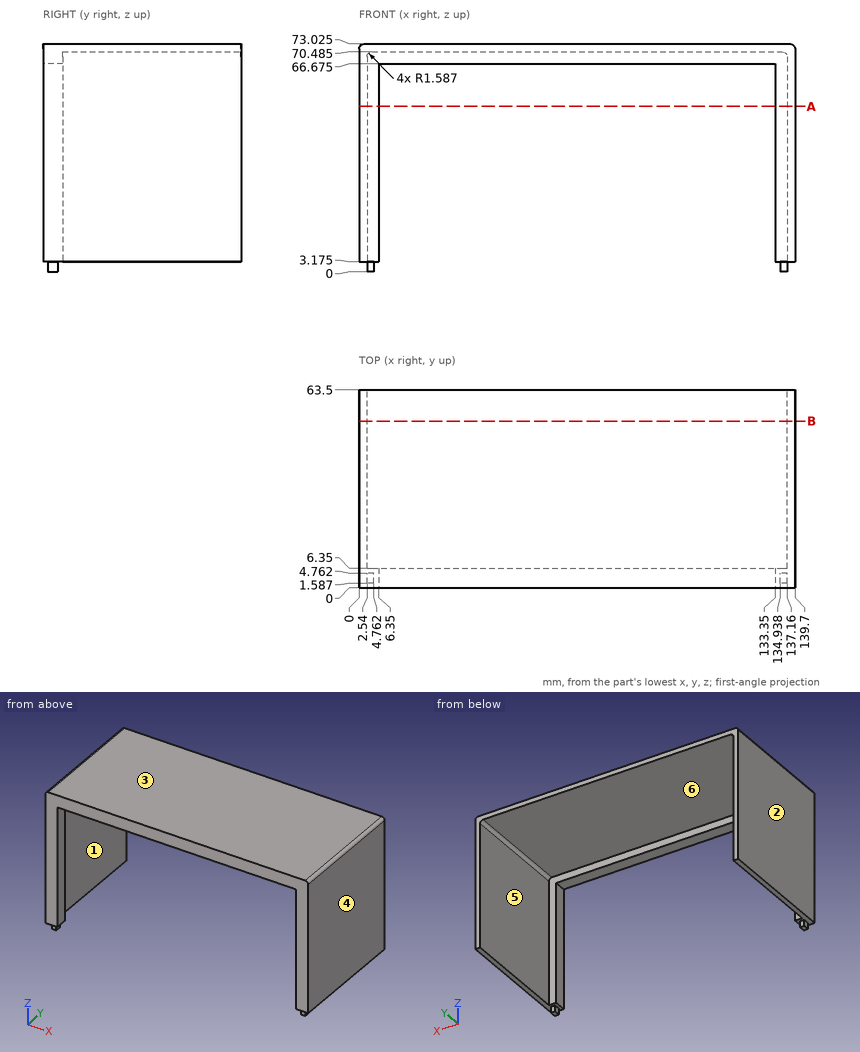
Job drawing, mm, ordinate dimensions from the low corner. One solid piece. A direction names the side the tool comes from. Round coordinates to 2 decimals unless told otherwise and drop trailing zeros. Loops run counter-clockwise (first coordinate to the right, second up) from the corner with the lowest first, then second, coordinate; pieces in that order, holes last.
Item 1: Drop flat-ended pins along their axis: P1, Ø1.6, axis at y = 3, z = 1.5, coming from the +X side; P2, Ø7, axis at x = 78.5, y = 3.5, coming from the -Z side (1 decimal); P3, Ø7, axis at x = 135.5, y = 41, coming from the -Z side (1 decimal). Give the stop position or say it passes through.
Item 2: Mould opens along X. For the marked faces 3, 4, 5 and 6 say: +X half, -X half, draft (parallel to the pull), parting line (faces both ways), or undercut.
Item 3: Cut at A-A, the plane z = 53. Give the cut face in (x, y), then the cut area to 3 significant figures.
Item 4: Drill centre lines: line 1 (X direction, y = 17.5, z = 43.5); line 2 (Z direction, x = 67, y = 52) (1 decimal); line 3 (Z direction, x = 23, y = 6) (1 decimal). Where is each one in solid material? Low to high.
Item 5: 3-axis set-ups, long thin cutter, end or side, ignore diameter. For the marked faces 1 and 2: which of +Z, -Z, +X, -X, +Y, -Y reach the whole face in a straight line?
Item 6: Cut at B-B, the plane y = 53.5. Give the cut face in (x, z) (1 decimal).
A:
1. P1: stops at x = 137.16
1. P2: stops at z = 66.7
1. P3: stops at z = 3.2
2. face 3: draft
2. face 4: +X half
2. face 5: undercut
2. face 6: undercut
3. outline: (0, 0) - (6.35, 0) - (6.35, 6.35) - (2.54, 6.35) - (2.54, 63.5) - (0, 63.5) - close; (133.35, 0) - (139.7, 0) - (139.7, 63.5) - (137.16, 63.5) - (137.16, 6.35) - (133.35, 6.35) - close
3. area: 371 mm2
4. line 1: x = 0 to 2.54, 137.16 to 139.7
4. line 2: z = 70.5 to 73
4. line 3: z = 66.7 to 73
5. face 1: -Z, +Y
5. face 2: +Z, -Z, -X, +Y, -Y
6. outline: (0, 3.2) - (2.5, 3.2) - (2.5, 68.9) arc R1.6 cw to (4.1, 70.5) - (135.6, 70.5) arc R1.6 cw to (137.2, 68.9) - (137.2, 3.2) - (139.7, 3.2) - (139.7, 71.4) arc R1.6 ccw to (138.1, 73) - (1.6, 73) arc R1.6 ccw to (0, 71.4) - close
